```python
from build123d import *

# Parameters (mm, degrees)
BOSS_EXTRUDE1_DEPTH = 15
FILLET1_R           = 3
CUT_EXTRUDE1_DEPTH  = 16.25
CHAMFER1_SIZE       = 0.4
CUT_EXTRUDE2_DEPTH  = 16.25
CHAMFER2_SIZE       = 2


with BuildPart() as part:
    # Sketch1 → Boss-Extrude1 (new body, symmetric)
    with BuildSketch(Plane(origin=(0, 0, 0), x_dir=(0, 0, -1), z_dir=(1, 0, 0))):
        Polygon((-7.625, 6.7), (-3.625, 6.7), (-3.625, 10.7), (-7.625, 10.7), (-7.625, 31.670562748), (1.404437252, 40.7), (7.625, 40.7), (7.625, 28.7), (6.375, 28.7), (4.375, 26.7), (4.375, 6.7), (7.625, 3.2), (7.625, -6.7), (-7.625, -6.7), align=None)
    extrude(amount=BOSS_EXTRUDE1_DEPTH, both=True)

    # Fillet1
    fillet1_edges = [part.edges().sort_by_distance(p)[0] for p in [
        (-15, 8.7, 3.625),
        (15, 8.7, 3.625),
    ]]
    fillet(fillet1_edges, radius=FILLET1_R)

    # Sketch2 → Cut-Extrude1 (cut, through all)
    with BuildSketch(Plane.XY.offset(7.625)):
        Polygon((-13.2, 2.9), (13.2, 2.9), (13.2, -2.55), (11.05, -4.7), (13.05, -6.7), (-13.05, -6.7), (-11.05, -4.7), (-13.2, -2.55), align=None)
    extrude(amount=-CUT_EXTRUDE1_DEPTH, mode=Mode.SUBTRACT)

    # Chamfer1
    chamfer1_edges = [part.edges().sort_by_distance(p)[0] for p in [
        (15, -1.75, -7.625),
        (-15, -1.75, -7.625),
        (-15, 0, 7.625),
        (0, 6.7, 7.625),
        (14.025, -6.7, -7.625),
        (14.025, -6.7, 7.625),
        (15, 0, 7.625),
        (-14.025, -6.7, -7.625),
        (-14.025, -6.7, 7.625),
        (-13.2, 0.175, -7.625),
        (13.2, 0.175, -7.625),
        (12.125, -3.625, -7.625),
        (12.05, -5.7, -7.625),
        (11.05, -4.7, 0),
        (-12.05, -5.7, -7.625),
        (-12.125, -3.625, -7.625),
        (-11.05, -4.7, 0),
        (-13.2, 0.175, 7.625),
        (-12.125, -3.625, 7.625),
        (-12.05, -5.7, 7.625),
        (12.05, -5.7, 7.625),
        (12.125, -3.625, 7.625),
        (13.2, 0.175, 7.625),
        (0, 2.9, 7.625),
    ]]
    chamfer(chamfer1_edges, length=CHAMFER1_SIZE)

    # Sketch3 → Cut-Extrude2 (cut, through all)
    with BuildSketch(Plane.XY.offset(7.625)):
        Polygon((-15, 31.670562748), (-9.786851972, 40.7), (-15, 40.7), align=None)
        Polygon((15, 31.670562748), (15, 40.7), (9.786851972, 40.7), align=None)
    extrude(amount=-CUT_EXTRUDE2_DEPTH, mode=Mode.SUBTRACT)

    # Chamfer2
    chamfer2_edges = [part.edges().sort_by_distance(p)[0] for p in [
        (0, 10.7, 7.625),
    ]]
    chamfer(chamfer2_edges, length=CHAMFER2_SIZE)


solid = part.part
```
Design review of the part built by this model. Coordinates are the model's own, in mm. A direction names the side the tool comes from. Coordinates: 2 decimals unless noted, no trailing zeros. Loops run counter-clockwise (first coordinate to the right, second up) from the corner with the lowest first, then second, coordinate; pieces in that order, holes last. Notation, with made-up numbers: M -17,5 L 35,5 A16 cw 35,29 Z; hole C -2,58 d6. An arc over 180 degrees is marked long. One line per question, with ' | ' between items.
(1) We need section C-C (z = -5). Give the boundary of the cut face in (x, y) (3 decimals).
Filled in:
outline: M -15,-6.7 L -13.05,-6.7 L -11.333,-4.983 L -11.333,-4.417 L -13.2,-2.55 L -13.2,2.9 L 13.2,2.9 L 13.2,-2.55 L 11.333,-4.417 L 11.333,-4.983 L 13.05,-6.7 L 15,-6.7 L 15,6.027 L -15,6.027 Z; M -15,27.325 L 15,27.325 L 15,31.671 L 9.787,40.7 L -9.787,40.7 L -15,31.671 Z
(2) For pin 1 Ø2 at (y, z) = (35, 2) entering from -X; pin 2 Ø1 at (x, z) = (2, -7) entering from -Y; pin 3 Ø6 at (x, z) = (-8.5, 3.5) entering from +Y, all flat-tipped, find the tip position at first contact; note any pin that passes through.
Filled in:
pin 1: stops at x = -13.66 | pin 2: stops at y = 2.9 | pin 3: stops at y = 38.8
(3) Machinability: for faces 1 (the face through (-12.451, -3.578, 7.422)), 2 (the face through (-12.2, -5.85, 0.1)), 3 (the face through (-12.3, -5.7, -7.4)), 4 (the face through (-12.3, -5.7, 7.4)), which of the approach directions +Z, -Z, +X, -X, +Y, -Y give a long, thin tool a straight path to every point of the face, cutting with its end or side? Answer none if there is none.
Filled in:
face 1: +Z | face 2: +Z, -Z, -Y | face 3: -Z, -Y | face 4: +Z, -Y
(4) We need section A-A (y = -1). Give the boundary of the cut face in (x, z) (3 decimals), and give its area (3 significant figures).
Filled in:
outline: M -15,-7.225 L -14.6,-7.625 L -13.6,-7.625 L -13.2,-7.225 L -13.2,7.225 L -13.6,7.625 L -14.6,7.625 L -15,7.225 Z; M 13.2,-7.225 L 13.6,-7.625 L 14.6,-7.625 L 15,-7.225 L 15,7.225 L 14.6,7.625 L 13.6,7.625 L 13.2,7.225 Z | area: 54.3 mm^2
(5) Wall thickness on probe 1 along X at (y, z) = (2.5, 3); probe 2 along Z at (x, y) = (3, 18) (3 decimals); probe 3 along Y at (x, z) = (7.5, -2.25): over which ranges is each line inside the solid? List them lowest first.
Filled in:
probe 1: x = -15 to -13.2, 13.2 to 15 | probe 2: z = -4.375 to 7.625 | probe 3: y = 2.9 to 40.7
(6) We need section B-B (x = -3). Give the boundary of the cut face in (y, z) (3 decimals), and give its area (3 significant figures).
Filled in:
outline: M 2.9,-7.625 L 3.2,-7.625 L 6.7,-4.375 L 26.7,-4.375 L 28.7,-6.375 L 28.7,-7.625 L 40.7,-7.625 L 40.7,-1.404 L 31.671,7.625 L 12.7,7.625 L 10.7,5.625 L 10.7,3.625 L 6.7,3.625 L 6.7,7.225 L 6.3,7.625 L 3.3,7.625 L 2.9,7.225 Z | area: 442 mm^2
(7) Draft analysis for pull direction X (two halves, no side actions). For faces 5 (the face through (12.936, 35.245, -1.588)), 6 (the face through (12.18, -5.83, 0.1)), 7 (the face through (0.21, 11.686, 6.611)), 8 (the face through (-13.01, 35.12, -1.59)), state which applies: released by +X, released by -X, zero draft, split by the parting line, or undercut.
Filled in:
face 5: released by +X | face 6: undercut | face 7: zero draft | face 8: released by -X
(8) We need section D-D (y = 10). Give the boundary of the cut face in (x, z) (3 decimals), and give its area (3 significant figures).
Filled in:
outline: M -15,-4.375 L 15,-4.375 L 15,0.625 A3 ccw 12,3.625 L -12,3.625 A3 ccw -15,0.625 Z | area: 236 mm^2
